from build123d import *

# Parameters (mm, degrees)
BOSS_EXTRU_1_DEPTH      = 10
ESQUISSE4_R             = 2
ENL_V_MAT_EXTRU_1_DEPTH = 25.779023387


with BuildPart() as part:
    # Esquisse3 → Boss.-Extru.1 (new body)
    with BuildSketch(Plane.XY):
        with BuildLine():
            Line((-15, 0), (15, 0))
            Line((15, 0), (15, 5))
            Line((15, 5), (8, 5))
            Line((8, 5), (8, 22))
            Line((8, 22), (1, 22))
            Line((1, 22), (1, 19.354101966))
            ThreePointArc((1, 19.354101966), (0, 12.5), (-1, 19.354101966))
            Line((-1, 19.354101966), (-1, 22))
            Line((-1, 22), (-8, 22))
            Line((-8, 22), (-8, 5))
            Line((-8, 5), (-15, 5))
            Line((-15, 5), (-15, 0))
        make_face()
    extrude(amount=BOSS_EXTRU_1_DEPTH)

    # Esquisse4 → Enlèv. mat.-Extru.1 (cut, through all)
    with BuildSketch(Plane(origin=(0, 5, 0), x_dir=(1, 0, 0), z_dir=(0, 1, 0))):
        with Locations(Location((11.5, -5, 0), (0, 0, 180))):
            Circle(ESQUISSE4_R)
        with Locations((-11.5, -5)):
            Circle(ESQUISSE4_R)
    extrude(amount=-ENL_V_MAT_EXTRU_1_DEPTH, mode=Mode.SUBTRACT)


solid = part.part
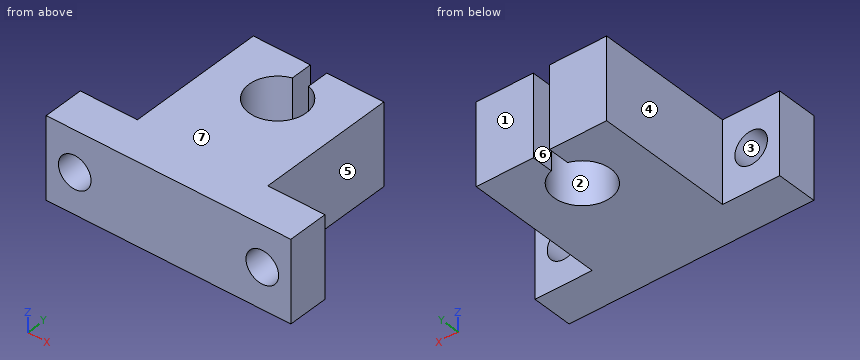
The listing builds one solid part. Answer for the finished solid, in the listing's coordinates (mm). Face numbers are marked on the shaded views. A direction names the side the tool comes from. Coordinates: 2 decimals unless noted, no trailing zeros. Order: outer loops, then holes, each group sorted by start corner. A loop starts at its lowest first (then second) coordinate and runs counter-clockwise, first axis right, second up.
Q1. A cutting plane is placed at A-A, the plane x = 11.5. Write down the section's boundary in (y, z), and give its area (3 significant figures).
Q2. For a pull along Y with two mould halves and no side action, classify the marked faces 1, 2 and 3 as pulls with the +Y half, pulls with the -Y half, needs draft (parallel to the pull), parting line crosses it, or undercut.
Q3. A cutting plane is placed at B-B, the plane y = 16. Write down the section's boundary in (x, z), and give its area (3 significant figures).
Q4. Consider line 1 (X direction, y = 16, z = 3.5); line 2 (Z direction, x = -11.5, y = 3.2); line 3 (Y direction, x = 0, z = 5.75). Determine where each line is inside the solid, lowest interval first.
Q5. A cutting plane is placed at C-C, the plane z = 5. Write down the section's boundary in (x, y), and give its area (3 significant figures).
Q6. Which of the six approach directions +Z, -Z, +X, -X, +Y, -Y give full straight-line access (tool end or side, diameter ignored) to the marked faces 4, 5, 6 and 7?
Q7. A cutting plane is placed at D-D, the plane y = 1.75. Write down the section's boundary in (x, z).
Q8. Given P1, Ø3, axis at x = -11.5, z = 5, coming from the +Y side; P2, Ø1, axis at y = 11, z = 7.5, coming from the +X side; P3, Ø5.5, axis at x = -11.5, z = 2.5, coming from the +Y side; P4, Ø3, axis at y = 20.5, z = 5, coming from the -X side, each flat-ended and moving along its own axis, determine where each tip first touches the part or whether it passes through.
Answers follow:
1. outline: (0, 0) - (5, 0) - (5, 3) - (0, 3) - close; (0, 7) - (5, 7) - (5, 10) - (0, 10) - close
1. area: 30.0 mm2
2. face 1: pulls with the +Y half
2. face 2: undercut
2. face 3: needs draft
3. outline: (-8, 0) - (-3.5, 0) - (-3.5, 10) - (-8, 10) - close; (3.5, 0) - (8, 0) - (8, 10) - (3.5, 10) - close
3. area: 90.0 mm2
4. line 1: x = -8 to -3.5, 3.5 to 8
4. line 2: z = 0 to 3, 7 to 10
4. line 3: y = 0 to 12.5
5. outline: (-15, 0) - (-13.5, 0) - (-13.5, 5) - (-15, 5) - close; (-9.5, 0) - (9.5, 0) - (9.5, 5) - (8, 5) - (8, 22) - (1, 22) - (1, 19.35) arc R3.5 cw (long way) to (-1, 19.35) - (-1, 22) - (-8, 22) - (-8, 5) - (-9.5, 5) - close; (13.5, 0) - (15, 0) - (15, 5) - (13.5, 5) - close
5. area: 338 mm2
6. face 4: +Z, -Z, -X, +Y
6. face 5: +Z, -Z, +X, +Y
6. face 6: +Z, -Z, +Y
6. face 7: +Z, +X, -X, +Y, -Y
7. outline: (-15, 0) - (15, 0) - (15, 10) - (-15, 10) - close; hole circle Ø4 at (-11.5, 5); hole circle Ø4 at (11.5, 5)
8. P1: passes through
8. P2: stops at x = 8
8. P3: stops at y = 5
8. P4: stops at x = -8
